Here's how the part is built. I have some questions about the finished solid (model axes, mm). A direction names the side the tool comes from. Coordinates: 2 decimals unless noted, no trailing zeros. Write each loop counter-clockwise with the first axis right and the second up, starting at its lowest first coordinate (ties: lowest second). Pieces come first, ordered by that corner, then holes. Notation, with made-up numbers: (-24, 65) - (-18, 65) arc R24 cw to (-18, 101) - close; hole circle Ø5 at (60.5, -19.75). An arc over 180 degrees is marked (long way). Answer in a Markdown table with one row per item. Add a question column.
Item 1: I'm going to push flat-ended pins straight in: pin 1 (2.5 mm diameter, centred on x = 1.5, y = 21, fed in from -Z); pin 2 (1 mm diameter, centred on x = 2.5, z = -18, fed in from +Y). Where does each tip first touch, or does it pass through?
Item 2: Imagine slicing it at A-A (z = -60). Please give me the cut outline in (x, y), plus the area to 3 significant figures.
Item 3: Imagine slicing it at C-C (x = 2.4). State how many separate pieces and enclosed holes the cut face has, plus the area to 3 significant figures.
Item 4: We'd pull the mould along Z, two halves only. Please class faces 6 (the face through (3, 23, -36.95)), 7 (the face through (2.5, 22.5, -6)), 8 (the face through (2, 0, -9)): +Z half, -Z half, draft (parallel to the pull), parting line (faces both ways), or undercut.
Item 5: Which directions (+Z, -Z, +X, -X, +Y, -Y) give clear straight access to the entire face, cutting with the end or side of a thin tool? Please do faces 1 (the face through (2, 16.55, -3)), 2 (the face through (3, 31, -43)), 3 (the face through (2, 0, -36)), 4 (the face through (3, 2, -51)), 5 (the face through (2, 45, -2)).
Item 6: Imagine slicing it at B-B (z = -71). Please give me the cut outline in (x, y), plus the area to 3 significant figures.
Item 7: If I drill on probe 1 along Z at (x, y) = (4, 24); probe 2 along Z at (x, y) = (0.5, 4.5); probe 3 along Y at (x, z) = (4.3, -39.5), over which ranges is the centre line in solid material (lowest first)? Write a range as from..to.
from build123d import *

# Parameters (mm, degrees)
SKETCH_1_W           = 91
SKETCH_1_H           = 45
EXTRUDE_1_DEPTH      = 5
SKETCH_7_W           = 24
SKETCH_7_H           = 9
CUT_EXTRUDE_3_DEPTH  = 10
FILLET_1_R           = 2
SKETCH_8_W           = 32
SKETCH_8_H           = 4
CUT_EXTRUDE_4_DEPTH  = 10
FILLET_2_R           = 2
SKETCH_9_W           = 5
SKETCH_9_H           = 17
CUT_EXTRUDE_5_DEPTH  = 5
SKETCH_14_R          = 1.55
SKETCH_14_R_2        = 1.482519405
CUT_EXTRUDE_9_DEPTH  = 10
SKETCH_10_R          = 1
CUT_EXTRUDE_6_DEPTH  = 10
SKETCH_12_R          = 1.6
CUT_EXTRUDE_7_DEPTH  = 10
CUT_EXTRUDE_8_DEPTH  = 10
SKETCH_15_W          = 10
SKETCH_15_H          = 5
CUT_EXTRUDE_10_DEPTH = 10
SKETCH_19_W          = 5
SKETCH_19_H          = 6.9
SKETCH_19_H_2        = 9.9
CUT_EXTRUDE_14_DEPTH = 5
SKETCH_16_R          = 1
CUT_EXTRUDE_11_DEPTH = 10
SKETCH_20_W          = 5.1
SKETCH_20_H          = 15.197667804
CUT_EXTRUDE_15_DEPTH = 10


with BuildPart() as part:
    # 스케치1 → 보스-돌출1 (new body)
    with BuildSketch(Plane(origin=(0, 0, 0), x_dir=(0, 0, -1), z_dir=(1, 0, 0))):
        with Locations((45.5, 22.5)):
            Rectangle(SKETCH_1_W, SKETCH_1_H)
    extrude(amount=EXTRUDE_1_DEPTH)

    # 스케치7 → 컷-돌출3 (cut)
    with BuildSketch(Plane(origin=(5, 0, 0), x_dir=(0, 0, -1), z_dir=(1, 0, 0))):
        with Locations((64, 22.5)):
            Rectangle(SKETCH_7_W, SKETCH_7_H)
    extrude(amount=-CUT_EXTRUDE_3_DEPTH, mode=Mode.SUBTRACT)

    # 필렛1
    fillet_1_edges = [part.edges().sort_by_distance(p)[0] for p in [
        (2.5, 18, -52),
        (2.5, 27, -52),
        (2.5, 27, -76),
        (2.5, 18, -76),
    ]]
    fillet(fillet_1_edges, radius=FILLET_1_R)

    # 스케치8 → 컷-돌출4 (cut)
    with BuildSketch(Plane(origin=(5, 0, 0), x_dir=(0, 0, -1), z_dir=(1, 0, 0))):
        with Locations((21, 43)):
            Rectangle(SKETCH_8_W, SKETCH_8_H)
    extrude(amount=-CUT_EXTRUDE_4_DEPTH, mode=Mode.SUBTRACT)

    # 필렛2
    fillet_2_edges = [part.edges().sort_by_distance(p)[0] for p in [
        (2.5, 41, -5),
        (2.5, 41, -37),
    ]]
    fillet(fillet_2_edges, radius=FILLET_2_R)

    # 스케치9 → 컷-돌출5 (cut)
    with BuildSketch(Plane.ZY):
        with Locations((-39.5, 23.5)):
            Rectangle(SKETCH_9_W, SKETCH_9_H)
    extrude(amount=-CUT_EXTRUDE_5_DEPTH, mode=Mode.SUBTRACT)

    # 스케치14 → 컷-돌출9 (cut)
    with BuildSketch(Plane(origin=(5, 0, 0), x_dir=(0, 0, -1), z_dir=(1, 0, 0))):
        with Locations((2.5, 10)):
            Circle(SKETCH_14_R)
        with Locations((2.5, 30)):
            Circle(SKETCH_14_R)
        with Locations((88.5, 35.067480595)):
            Circle(SKETCH_14_R_2)
        with Locations((88.5, 10)):
            Circle(SKETCH_14_R)
    extrude(amount=-CUT_EXTRUDE_9_DEPTH, mode=Mode.SUBTRACT)

    # 스케치10 → 컷-돌출6 (cut)
    with BuildSketch(Plane(origin=(5, 0, 0), x_dir=(0, 0, -1), z_dir=(1, 0, 0))):
        with Locations((42, 31)):
            Circle(SKETCH_10_R)
        with Locations((42, 16)):
            Circle(SKETCH_10_R)
        with Locations((37, 16)):
            Circle(SKETCH_10_R)
        with Locations((37, 31)):
            Circle(SKETCH_10_R)
    extrude(amount=-CUT_EXTRUDE_6_DEPTH, mode=Mode.SUBTRACT)

    # 스케치12 → 컷-돌출7 (cut)
    with BuildSketch(Plane(origin=(5, 0, 0), x_dir=(0, 0, -1), z_dir=(1, 0, 0))):
        with Locations((2.5, 30)):
            Circle(SKETCH_12_R)
        with Locations((2.5, 10)):
            Circle(SKETCH_12_R)
        with Locations((88.5, 35)):
            Circle(SKETCH_12_R)
        with Locations((88.5, 10)):
            Circle(SKETCH_12_R)
    extrude(amount=-CUT_EXTRUDE_7_DEPTH, mode=Mode.SUBTRACT)

    # 스케치13 → 컷-돌출8 (cut)
    with BuildSketch(Plane(origin=(5, 0, 0), x_dir=(0, 0, -1), z_dir=(1, 0, 0))):
        with BuildLine():
            Line((18.45, 0), (18.45, 6))
            Line((18.45, 6), (17.250192706, 6))
            ThreePointArc((17.250192706, 6), (15.841386702, 7.391138254), (17.232524956, 8.799944258))
            Line((17.232524956, 8.799944258), (18.45, 8.799944258))
            Line((18.45, 8.799944258), (18.45, 10))
            ThreePointArc((18.45, 10), (20, 11.55), (21.55, 10))
            Line((21.55, 10), (21.55, 8.799872773))
            Line((21.55, 8.799872773), (22.749807294, 8.799872773))
            ThreePointArc((22.749807294, 8.799872773), (24.117188413, 7.432491654), (22.749807294, 6.065110535))
            Line((22.749807294, 6.065110535), (21.55, 6.065110535))
            Line((21.55, 6.065110535), (21.55, 0))
            Line((21.55, 0), (18.45, 0))
        make_face()
        with BuildLine():
            Line((72.55, 0), (72.55, 6.065110535))
            Line((72.55, 6.065110535), (73.749807294, 6.065110535))
            ThreePointArc((73.749807294, 6.065110535), (75.117188413, 7.432491654), (73.749807294, 8.799872773))
            Line((73.749807294, 8.799872773), (72.55, 8.799872773))
            Line((72.55, 8.799872773), (72.55, 10))
            ThreePointArc((72.55, 10), (71, 11.55), (69.45, 10))
            Line((69.45, 10), (69.45, 8.799944258))
            Line((69.45, 8.799944258), (68.232524956, 8.799944258))
            ThreePointArc((68.232524956, 8.799944258), (66.841386702, 7.391138254), (68.250192706, 6))
            Line((68.250192706, 6), (69.45, 6))
            Line((69.45, 6), (69.45, 0))
            Line((69.45, 0), (72.55, 0))
        make_face()
    extrude(amount=-CUT_EXTRUDE_8_DEPTH, mode=Mode.SUBTRACT)

    # 스케치15 → 컷-돌출10 (cut)
    with BuildSketch(Plane(origin=(5, 0, 0), x_dir=(0, 0, -1), z_dir=(1, 0, 0))):
        with Locations((56, 2.5)):
            Rectangle(SKETCH_15_W, SKETCH_15_H)
    extrude(amount=-CUT_EXTRUDE_10_DEPTH, mode=Mode.SUBTRACT)

    # 스케치19 → 컷-돌출14 (cut)
    with BuildSketch(Plane.ZY):
        with Locations((-2.5, 20)):
            Rectangle(SKETCH_19_W, SKETCH_19_H)
        with Locations((-88.5, 22.5)):
            Rectangle(SKETCH_19_W, SKETCH_19_H_2)
    extrude(amount=-CUT_EXTRUDE_14_DEPTH, mode=Mode.SUBTRACT)

    # 스케치16 → 컷-돌출11 (cut)
    with BuildSketch(Plane.ZY):
        with Locations((-60, 5)):
            Circle(SKETCH_16_R)
        with Locations((-52, 5)):
            Circle(SKETCH_16_R)
        with Locations((-86, 26.45)):
            Circle(SKETCH_16_R)
        with Locations((-86, 18.55)):
            Circle(SKETCH_16_R)
        with Locations((-5, 22.45)):
            Circle(SKETCH_16_R)
        with Locations((-5, 17.55)):
            Circle(SKETCH_16_R)
    extrude(amount=-CUT_EXTRUDE_11_DEPTH, mode=Mode.SUBTRACT)

    # 스케치20 → 컷-돌출15 (cut)
    with BuildSketch(Plane(origin=(5, 0, 0), x_dir=(0, 0, -1), z_dir=(1, 0, 0))):
        with Locations((39.5, 23.598833902)):
            Rectangle(SKETCH_20_W, SKETCH_20_H)
    extrude(amount=-CUT_EXTRUDE_15_DEPTH, mode=Mode.SUBTRACT)


solid = part.part
Here are the results:
| question | item | result |
|---|---|---|
| 1 | pin 1 | stops at z = -86 |
| 1 | pin 2 | stops at y = 41 |
| 2 | outline | (0, 6) - (5, 6) - (5, 18) - (0, 18) - close; (0, 27) - (5, 27) - (5, 45) - (0, 45) - close |
| 2 | area | 150 mm2 |
| 3 | separate pieces | 1 |
| 3 | enclosed holes | 6 |
| 3 | area | 3,390 mm2 |
| 4 | face 6 | undercut |
| 4 | face 7 | +Z half |
| 4 | face 8 | draft |
| 5 | face 1 | +Z, +X, -X |
| 5 | face 2 | +X, -X |
| 5 | face 3 | +Z, -Z, +X, -X, -Y |
| 5 | face 4 | +X, -X, -Y |
| 5 | face 5 | +Z, -Z, +X, -X, +Y |
| 6 | outline | (0, 11.55) - (5, 11.55) - (5, 18) - (0, 18) - close; (0, 27) - (5, 27) - (5, 45) - (0, 45) - close |
| 6 | area | 122 mm2 |
| 7 | probe 1 | z = -86..-76, -52..-42.05, -36.95..0 |
| 7 | probe 2 | z = -91..-72.55, -69.45..-61, -51..-21.55, -18.45..0 |
| 7 | probe 3 | y = 0..15, 32..45 |
